Can you work these out from the model? Positions are in its coordinate system, mm. Coordinates: 2 decimals unless noted, no trailing zeros. Loops run counter-clockwise (first coordinate to the right, second up) from the corner with the lowest first, then second, coordinate; pieces in that order, holes last. Notation, with made-up numbers: M 46.5,27.5 L 85.5,27.5 A24 ccw 85.5,62.5 Z; hole C 19,29.25 d9. An arc over 180 degrees is marked long. Answer as a JSON object with one key per item and string values. Group by question number.
Item 1: Suppose I cut it at D-D (y = 2.85). Count the separate pieces of the cut face and the enclosed holes in it, then the cut area to 3 significant figures.
Item 2: Suppose I cut it at C-C (x = -50.8). Write out the boundary of the cut face in (y, z) (1 decimal).
Item 3: Suppose I cut it at B-B (x = -12.7). Write out the boundary of the cut face in (y, z) (1 decimal).
Item 4: If I drill on line 1 (Z direction, x = -12.7, y = 1.35) (3 decimals); line 2 (X direction, y = 3.25, z = -6); line 3 (Z direction, x = -10.5, y = 1.7), over which ranges is the centre line in solid material (lowest first)?
Item 5: I'm going to push flat-ended pins straight in: pin 1 Ø3 at (x, z) = (-12.7, -30.988) entering from +Y; pin 2 Ø1.5 at (y, z) = (3, -16.5) entering from +X; pin 3 Ø2.5 at (x, y) = (-31.5, 1.5) entering from -Z; pin 4 Ø0.7 at (y, z) = (2, -24.5) entering from -X. Where does each tip first touch, or does it pass through?
Item 6: Suppose I cut it at A-A (x = -63.5). Write out the boundary of the cut face in (y, z) (1 decimal), then the cut area to 3 significant figures.
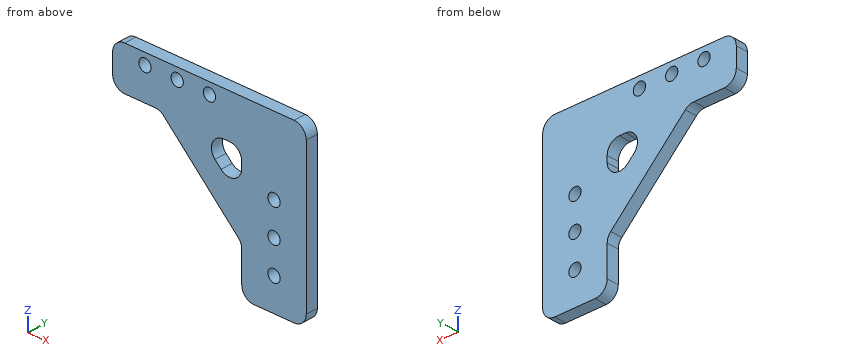
Autodesk Inventor part; units mm, degrees
ref_plane "YZ Plane" through (0, 0, 0) normal (1, 0, 0) x (0, 1, 0)
ref_plane "XZ Plane" through (0, 0, 0) normal (0, 1, 0) x (-1, 0, 0)
ref_plane "XY Plane" through (0, 0, 0) normal (0, 0, 1) x (1, 0, 0)
sketch "Sketch1" plane through (0, 0, 0) normal (0, 1, 0) x (-1, 0, 0)
  line L0 (0, -4.7625) -> (0, -64.3255)
  line L1 (4.7625, -69.088) -> (20.6375, -69.088)
  line L2 (76.2, -13.5255) -> (76.2, -4.7625)
  line L3 (71.4375, 0) -> (4.7625, 0)
  circle A0 centre (12.7, -30.988) radius 2.413
  arc A1 (4.7625, 0) -> (0, -4.7625) centre (4.7625, -4.7625) ccw
  circle A2 centre (12.7, -43.688) radius 2.413
  circle A3 centre (12.7, -56.388) radius 2.413
  circle A4 centre (38.1, -5.588) radius 2.413
  circle A5 centre (50.8, -5.588) radius 2.413
  circle A6 centre (63.5, -5.588) radius 2.413
  line L4 (14.4062, -54.6818) -> (61.7938, -7.2942) construction
  line L5 (26.7949, -49.0283) -> (56.1403, -19.6829)
  line L6 (33.5301, -28.8227) -> (35.9347, -26.4181)
  line L7 (25.4, -69.088) -> (25.4, -18.288) construction
  line L8 (76.2, -18.288) -> (25.4, -18.288) construction
  line L9 (25.4, -52.3959) -> (25.4, -64.3255)
  line L10 (71.4375, -18.288) -> (59.5079, -18.288)
  arc A7 (71.4375, -18.288) -> (76.2, -13.5255) centre (71.4375, -13.5255) ccw
  arc A8 (76.2, -4.7625) -> (71.4375, 0) centre (71.4375, -4.7625) ccw
  arc A9 (20.6375, -69.088) -> (25.4, -64.3255) centre (20.6375, -64.3255) ccw
  arc A10 (0, -64.3255) -> (4.7625, -69.088) centre (4.7625, -64.3255) ccw
  line L11 (32.5671, -18.288) -> (30.1625, -18.288)
  line L12 (25.4, -25.4551) -> (25.4, -23.0505)
  arc A11 (59.5079, -18.288) -> (56.1403, -19.6829) centre (59.5079, -23.0505) ccw
  arc A12 (26.7949, -49.0283) -> (25.4, -52.3959) centre (30.1625, -52.3959) ccw
  arc A13 (35.9347, -26.4181) -> (32.5671, -18.288) centre (32.5671, -23.0505) ccw
  arc A14 (25.4, -25.4551) -> (33.5301, -28.8227) centre (30.1625, -25.4551) ccw
  arc A15 (30.1625, -18.288) -> (25.4, -23.0505) centre (30.1625, -23.0505) ccw
  point P0 (0, 0)
  point P1 (0, 7.112)
  point P2 (0, -69.088)
  point P3 (25.4, -50.4232)
  point P4 (57.5352, -18.288)
  point P5 (25.4, -36.9528)
  point P6 (44.0648, -18.288)
  dimension "d0" = 76.2
  dimension "d1" = 4.826
  dimension "d2" = 4.7625
  dimension "d3" = 12.7
  dimension "d4" = 12.7
  dimension "d5" = 12.7
  dimension "d7" = 12.7
  dimension "d8" = 12.7
  dimension "d9" = 38.1
  dimension "d10" = 25.4
  dimension "d11" = 4.7625
  dimension "d12" = 4.7625
  dimension "d13" = 4.7625
  dimension "d14" = 4.7625
  dimension "d15" = 4.7625
  dimension "d16" = 18.288
  dimension "d17" = 25.4
  dimension "d18" = 76.2
  dimension "d19" = 12.7
  dimension "d20" = 38.1
extrude "Extrusion1" add sketch "Sketch1" along normal blind 4.7625
thread "Thread2"
thread "Thread3"
thread "Thread4"
thread "Thread5"
thread "Thread6"
thread "Thread7"
sketch "Sketch2" plane through (0, 4.7625, 0) normal (0, 1, 0) x (1, 0, 0)
  line L0 (-71.4375, 0) -> (-4.7625, 0)
  line L1 (-76.2, 1.27) -> (0, 1.27)
  line L2 (-76.2, 13.5255) -> (-76.2, 4.7625)
  line L3 (0, 4.7625) -> (0, 64.3255)
  line L4 (0, 1.27) -> (0, 0)
  line L5 (0, 0) -> (-76.2, 0)
  line L6 (-76.2, 0) -> (-76.2, 1.27)
  dimension "d37" = 1.27
extrude "Extrusion2" cut sketch "Sketch2" against normal through all
fillet "Fillet1" radius 4.7752 2 edges at (-74.6754, 2.3813, -1.27) (-1.5246, 2.3813, -1.27)
properties part number "ELEV_012_SUPBRK2_THRD" material "Aluminum 6061"
From the geometry:
{
 "1": {"separate pieces": "1", "enclosed holes": "7", "area": "2,860 mm2"},
 "2": {"outline": "M 0,-25 L 4.8,-25 L 4.8,-8 L 0,-8 Z; M 0,-3.2 L 4.8,-3.2 L 4.8,-1.3 L 0,-1.3 Z"},
 "3": {"outline": "M 0,-69.1 L 4.8,-69.1 L 4.8,-58.8 L 0,-58.8 Z; M 0,-54 L 4.8,-54 L 4.8,-46.1 L 0,-46.1 Z; M 0,-41.3 L 4.8,-41.3 L 4.8,-33.4 L 0,-33.4 Z; M 0,-28.6 L 4.8,-28.6 L 4.8,-1.3 L 0,-1.3 Z"},
 "4": {"line 1": "-69.088 to -58.801, -53.975 to -46.101, -41.275 to -33.401, -28.575 to -1.27", "line 2": "-76.2 to -65.88, -61.12 to -53.18, -48.42 to -40.48, -35.72 to 0", "line 3": "-69.09 to -57.38, -55.4 to -44.68, -42.7 to -31.98, -30 to -1.27"},
 "5": {"pin 1": "through", "pin 2": "x = 0", "pin 3": "z = -45.57", "pin 4": "x = -51.67"},
 "6": {"outline": "M 0,-18.3 L 4.8,-18.3 L 4.8,-8 L 0,-8 Z; M 0,-3.2 L 4.8,-3.2 L 4.8,-1.3 L 0,-1.3 Z", "area": "58.1 mm2"}
}
